Here's the drawing with two shaded views (mm, measured from the low corner). I have some questions. A direction names the side the tool comes from. Give positions to 0.01 mm unless a question says otherwise; leave off trailing zeros. Loops run counter-clockwise (first coordinate to the right, second up) from the corner with the lowest first, then second, coordinate; pieces in that order, holes last. Notation, with made-up numbers: (70.25, 78) -> (124.25, 78) arc R16 cw to (124.25, 87) -> close; hole circle Ø1 at (-32.5, -15.75). An arc over 180 degrees is marked (long way). Write each question's results on one line, items separated by ' | '. Start each with the question number.
Q1. If we section it at A-A, the plane y = 35: List the corners of the cut face in (x, z) for me, plus the area to 3 significant figures.
Q2. If we section it at B-B, the plane z = 55.5: List the corners of the cut face in (x, y) for me.
Q3. We'd pull the mould along Y, two halves only. Please class the marked faces 5, 6, 7 and 8: released by +Y, released by -Y, zero draft, split by the parting line, or undercut.
Q4. If I drill on line 1 along X through (y, z) = (85.5, 71.5); line 2 along Z through (x, y) = (127.5, 94.5); line 3 along Y through (x, z) = (75.5, 93.5), over which ranges is the centre line in solid material (lowest first)?
Q5. If we section it at D-D, the plane z = 14.5: List the corners of the cut face in (x, y) for me.
Q6. If we section it at C-C, the plane y = 95.5: List the corners of the cut face in (x, z) for me, plus the area to 3 significant figures.
Q7. Which directions (+Z, -Z, +X, -X, +Y, -Y) give clear straight access to the entire face, cutting with the end or side of a thin tool? Please do the marked faces 1, 2, 3 and 4.
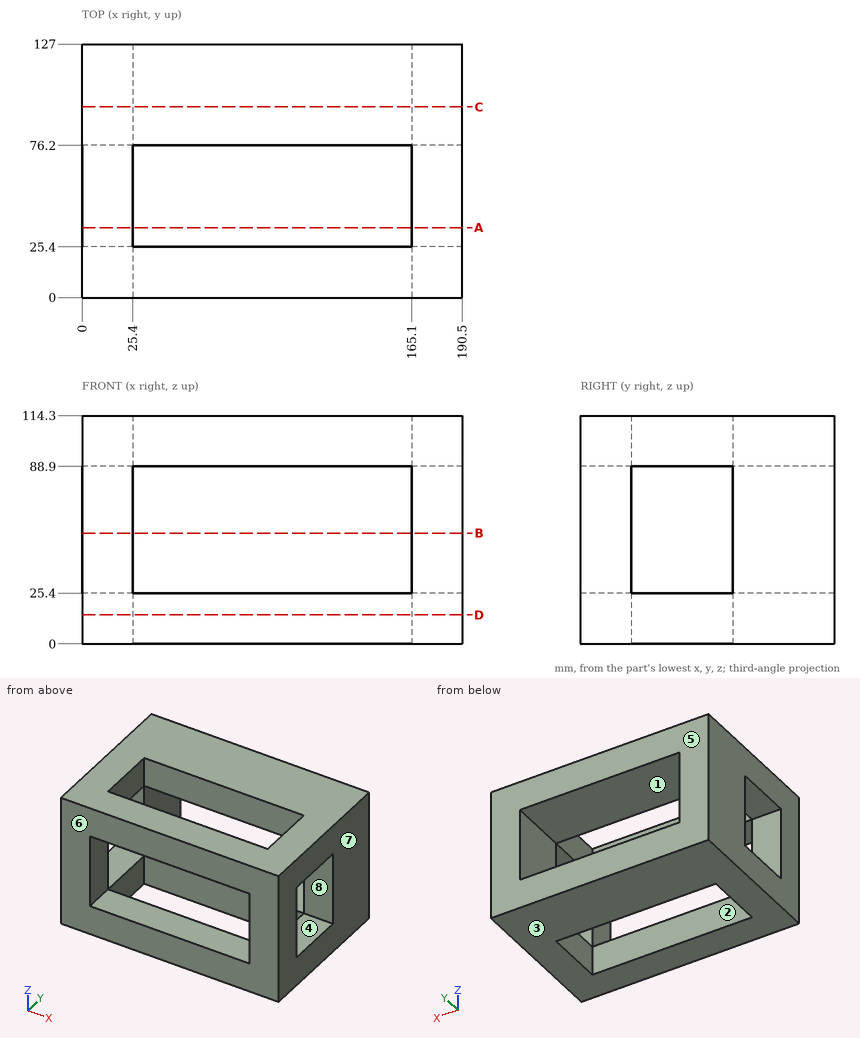
Final values:
1) outline: (0, 0) -> (25.4, 0) -> (25.4, 25.4) -> (0, 25.4) -> close; (0, 88.9) -> (25.4, 88.9) -> (25.4, 114.3) -> (0, 114.3) -> close; (165.1, 0) -> (190.5, 0) -> (190.5, 25.4) -> (165.1, 25.4) -> close; (165.1, 88.9) -> (190.5, 88.9) -> (190.5, 114.3) -> (165.1, 114.3) -> close | area: 2,580 mm²
2) outline: (0, 0) -> (25.4, 0) -> (25.4, 25.4) -> (0, 25.4) -> close; (0, 76.2) -> (25.4, 76.2) -> (25.4, 127) -> (0, 127) -> close; (165.1, 0) -> (190.5, 0) -> (190.5, 25.4) -> (165.1, 25.4) -> close; (165.1, 76.2) -> (190.5, 76.2) -> (190.5, 127) -> (165.1, 127) -> close
3) face 5: released by +Y | face 6: released by -Y | face 7: zero draft | face 8: undercut
4) line 1: x = 0 to 25.4, 165.1 to 190.5 | line 2: z = 0 to 25.4, 88.9 to 114.3 | line 3: y = 0 to 25.4, 76.2 to 127
5) outline: (0, 0) -> (190.5, 0) -> (190.5, 127) -> (0, 127) -> close; hole (25.4, 25.4) -> (165.1, 25.4) -> (165.1, 76.2) -> (25.4, 76.2) -> close
6) outline: (0, 0) -> (190.5, 0) -> (190.5, 114.3) -> (0, 114.3) -> close; hole (25.4, 25.4) -> (165.1, 25.4) -> (165.1, 88.9) -> (25.4, 88.9) -> close | area: 12,900 mm²
7) face 1: +Y, -Y | face 2: +Z, -Z | face 3: -Z, +X, -X, +Y, -Y | face 4: +X, -X
